```python
from build123d import *

# Parameters (mm, degrees)
SKETCH1_R                            = 14
BOSS_EXTRUDE1_DEPTH                  = 3
SKETCH2_R                            = 6.95
BOSS_EXTRUDE2_DEPTH                  = 1.5
SKETCH3_R                            = 3
CUT_EXTRUDE1_DEPTH                   = 21.303940504
SKETCH4_R                            = 7
SKETCH4_R_2                          = 3
SHAFT_HUB_COLLAR_L11_DEPTH           = 11
SKETCH5_R                            = 1.4
FLANGE_FOUR_D2P8_PCD22_DEPTH         = 3.01
DIN1481_D2_CROSS_PIN_HOLE_DEPTH      = 23.649503306
DIN1481_D2_CROSS_PIN_HOLE_DEPTH_BACK = 23.649503306
SKETCH6_R                            = 1


with BuildPart() as part:
    # Sketch1 → Boss-Extrude1 (new body)
    with BuildSketch(Plane.XY):
        Circle(SKETCH1_R)
    extrude(amount=BOSS_EXTRUDE1_DEPTH)

    # Sketch2 → Boss-Extrude2 (add)
    with BuildSketch(Plane.XY.offset(3)):
        Circle(SKETCH2_R)
    extrude(amount=BOSS_EXTRUDE2_DEPTH)

    # Sketch3 → Cut-Extrude1 (cut, through all)
    with BuildSketch(Plane.XY.offset(4.5)):
        Circle(SKETCH3_R)
    extrude(amount=-CUT_EXTRUDE1_DEPTH, mode=Mode.SUBTRACT)

    # Sketch4 → Shaft_Hub_Collar_L11 (add)
    with BuildSketch(Plane.XY):
        Circle(SKETCH4_R)
        Circle(SKETCH4_R_2, mode=Mode.SUBTRACT)
    extrude(amount=-SHAFT_HUB_COLLAR_L11_DEPTH)

    # Sketch5 → Flange_Four_D2p8_PCD22 (cut)
    with BuildSketch(Plane(origin=(0, 0, 0), x_dir=(-1, 0, 0), z_dir=(0, 0, -1))):
        with Locations((-7.778174593, 7.778174593)):
            Circle(SKETCH5_R)
        with Locations((7.778174593, 7.778174593)):
            Circle(SKETCH5_R)
        with Locations((7.778174593, -7.778174593)):
            Circle(SKETCH5_R)
        with Locations((-7.778174593, -7.778174593)):
            Circle(SKETCH5_R)
    extrude(amount=-FLANGE_FOUR_D2P8_PCD22_DEPTH, mode=Mode.SUBTRACT)

    # Sketch6 → DIN1481_D2_Cross_Pin_Hole (cut, two sides: drawn at the far end of the back side and taken through both)
    with BuildSketch(Plane(origin=(0, 0, 0), x_dir=(0, 0, -1), z_dir=(1, 0, 0)).offset(-DIN1481_D2_CROSS_PIN_HOLE_DEPTH_BACK)):
        with Locations((6, 0)):
            Circle(SKETCH6_R)
    extrude(amount=DIN1481_D2_CROSS_PIN_HOLE_DEPTH + DIN1481_D2_CROSS_PIN_HOLE_DEPTH_BACK, mode=Mode.SUBTRACT)


solid = part.part
```
CAD build for the part. Positions are in the model's coordinates, mm. A direction names the side the tool comes from. Round coordinates to 2 decimals unless told otherwise and drop trailing zeros. Order: outer loops, then holes, each group sorted by start corner. A loop starts at its lowest first (then second) coordinate and runs counter-clockwise, first axis right, second up. Notation, with made-up numbers: (5.5, -15.5) - (62.5, -15.5) arc R18 ccw to (62.5, -10.5) - close; hole circle Ø8 at (61.5, -17.75). An arc over 180 degrees is marked (long way). Answer as CSV lines item,"result". Start each with the question number.
1. Drill centre lines: L1, parallel to Y at x = 0, z = 0.25; L2, parallel to Z at x = 4.2, y = 0; L3, parallel to Y at x = 0, z = -0.5. Where is each one in solid material? Low to high. Write a range as [from, to].
2. Saw through at A-A, the plane x = 0. Write the cut outline in (y, z).
3. Pull direction Y, two halves, no side cores. Call faces 1 (the face through (-9.071, -8.314, 1.479)), 2 (the face through (-1.507, -6.785, 3.74)), 3 (the face through (-6.4, 3.3, 3)), 4 (the face through (9.177, 7.84, 1.479)): +Y half, -Y half, draft (parallel to the pull), parting line (faces both ways), or undercut.
4. Pin check, flat tips, straight feed: pin 1 (4 mm diameter, centred on y = 6, z = 1, fed in from -X); pin 2 (2 mm diameter, centred on y = 8.5, z = 0, fed in from -X); pin 3 (1 mm diameter, centred on x = -11, y = 5.5, fed in from +Z); pin 4 (3.5 mm diameter, centred on x = 0, y = 0, fed in from -Z). Stop position of each tip, or through.
5. Saw through at B-B, the plane y = 0. Write the cut outline in (x, z), and give its area (3 significant figures).
6. Tool access for faces 5 (the face through (6.677, 2.103, -5.423)), 6 (the face through (12.932, -5.362, 1.479)): list every direction of +Z, -Z, +X, -X, +Y, -Y with a clear straight run to the whole face (end or side of a thin tool).
7. Saw through at C-C, the plane x = 8.5. Write the cut outline in (y, z), and give its area (3 significant figures).
8. Saw through at D-D, the plane z = -6. Write the cut outline in (x, y), and give its area (3 significant figures).
Model answer:
1,L1,"y = [-14, -3], [3, 14]"
1,L2,"z = [-11, -7], [-5, 4.5]"
1,L3,"y = [-7, -3], [3, 7]"
2,outline,"(-14, 0) - (-7, 0) - (-7, -11) - (-3, -11) - (-3, 4.5) - (-6.95, 4.5) - (-6.95, 3) - (-14, 3) - close; (3, -11) - (7, -11) - (7, 0) - (14, 0) - (14, 3) - (6.95, 3) - (6.95, 4.5) - (3, 4.5) - close"
3,face 1,"undercut"
3,face 2,"parting line"
3,face 3,"draft"
3,face 4,"undercut"
4,pin 1,"stops at x = -13.42"
4,pin 2,"stops at x = -11.82"
4,pin 3,"stops at z = 3"
4,pin 4,"passes through"
5,outline,"(-14, 0) - (-7, 0) - (-7, -5) - (-3, -5) - (-3, 4.5) - (-6.95, 4.5) - (-6.95, 3) - (-14, 3) - close; (-7, -11) - (-3, -11) - (-3, -7) - (-7, -7) - close; (3, -11) - (7, -11) - (7, -7) - (3, -7) - close; (3, -5) - (7, -5) - (7, 0) - (14, 0) - (14, 3) - (6.95, 3) - (6.95, 4.5) - (3, 4.5) - close"
5,area,"150 mm²"
6,face 5,"-Z"
6,face 6,"+Z, -Z"
7,outline,"(-11.12, 0) - (-8.98, 0) - (-8.98, 3) - (-11.12, 3) - close; (-6.58, 0) - (6.58, 0) - (6.58, 3) - (-6.58, 3) - close; (8.98, 0) - (11.12, 0) - (11.12, 3) - (8.98, 3) - close"
7,area,"52.4 mm²"
8,outline,"(-6.93, -1) arc R7 ccw to (6.93, -1) - (2.83, -1) arc R3 cw to (-2.83, -1) - close; (-6.93, 1) - (-2.83, 1) arc R3 cw to (2.83, 1) - (6.93, 1) arc R7 ccw to start"
8,area,"110 mm²"
